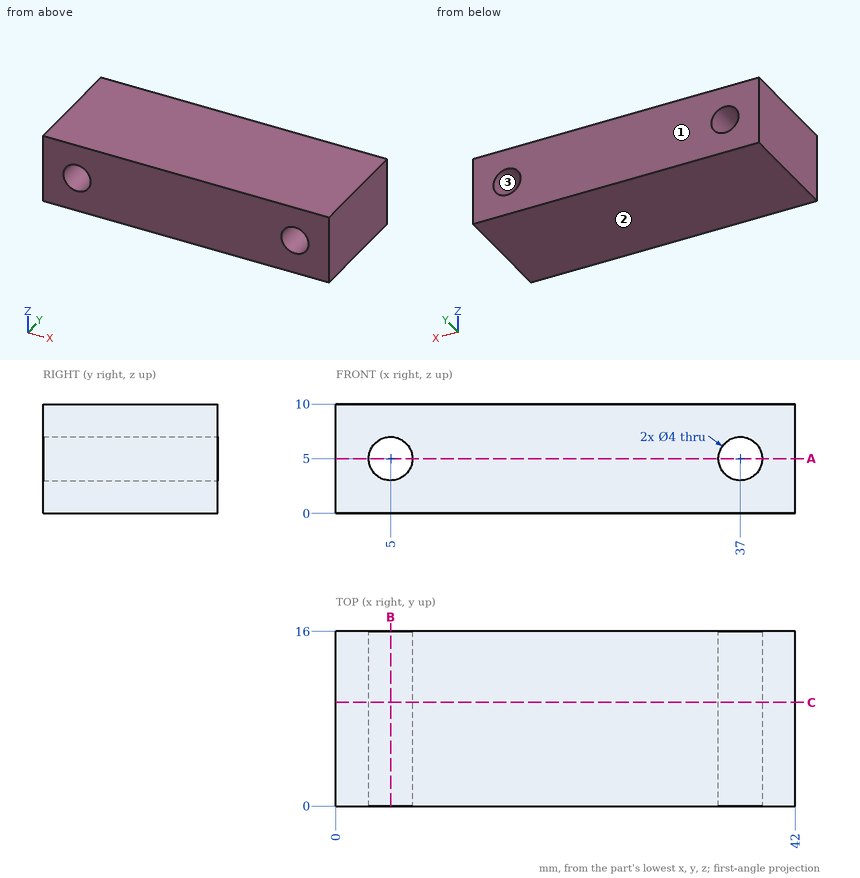
The figure shows three views and two pictorial views of one solid part (mm, origin at its lowest corner). Answer the questions. Coordinates: 2 decimals unless noted, no trailing zeros. Loops run counter-clockwise (first coordinate to the right, second up) from the corner with the lowest first, then second, coordinate; pieces in that order, holes last.
(1) The part is cut by section A-A (z = 5). Determine the outline of the cut face in (x, y), and give its area (3 significant figures).
Solution:
outline: (0, 0) - (3, 0) - (3, 16) - (0, 16) - close; (7, 0) - (35, 0) - (35, 16) - (7, 16) - close; (39, 0) - (42, 0) - (42, 16) - (39, 16) - close
area: 544 mm2
(2) The mould has two halves that part along Z. Classify the marked faces 1, 2 and 3: released by +Z, released by -Z, zero draft, split by the parting line, or undercut.
Solution:
face 1: zero draft
face 2: released by -Z
face 3: undercut
(3) The part is cut by section B-B (x = 5). Determine the outline of the cut face in (y, z), and give its area (3 significant figures).
Solution:
outline: (0, 0) - (16, 0) - (16, 3) - (0, 3) - close; (0, 7) - (16, 7) - (16, 10) - (0, 10) - close
area: 96.0 mm2
(4) Consider line 1 along X through (y, z) = (6, 5); line 2 along X through (y, z) = (11.75, 6); line 3 along Z through (x, y) = (5, 4.75). Determine where each line is inside the solid, lowest interval first.
Solution:
line 1: x = 0 to 3, 7 to 35, 39 to 42
line 2: x = 0 to 3.27, 6.73 to 35.27, 38.73 to 42
line 3: z = 0 to 3, 7 to 10
(5) A flat-ended cylindrical pin translates along its axis: pin 1 Ø1.5 at (x, z) = (36.5, 6) entering from -Y. Find the tip coordinate at first contact, or state that the pin passes through.
Solution:
pin 1: passes through
(6) The part is cut by section C-C (y = 9.5). Determine the outline of the cut face in (x, z), and give its area (3 significant figures).
Solution:
outline: (0, 0) - (42, 0) - (42, 10) - (0, 10) - close; hole circle Ø4 at (5, 5); hole circle Ø4 at (37, 5)
area: 395 mm2
